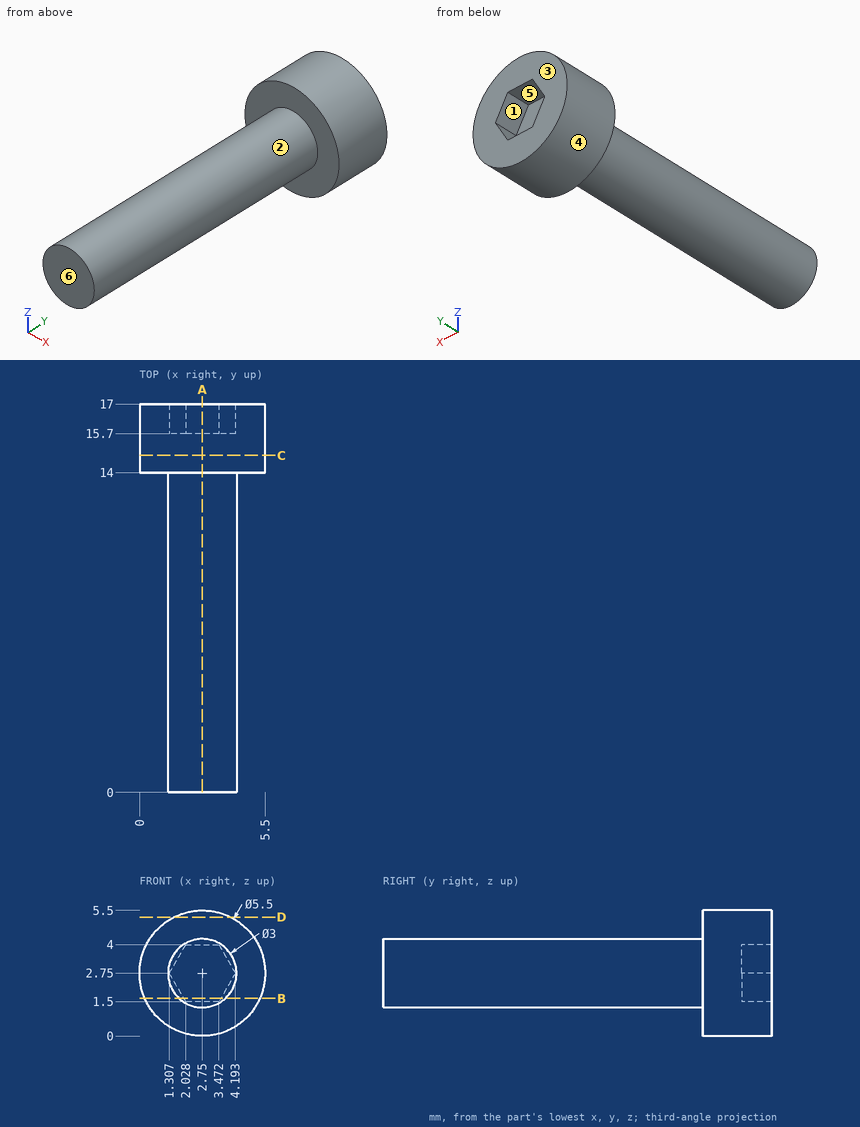
Answer from the drawing. Dimensions are ordinates in mm from the lowest x, y and z of the part. A direction names the side the tool comes from. Coordinates: 2 decimals unless noted, no trailing zeros. Order: outer loops, then holes, each group sorted by start corner. A loop starts at its lowest first (then second) coordinate and runs counter-clockwise, first axis right, second up. Notation, with made-up numbers: M -9.5,85 L 8.5,85 A24 ccw 8.5,122 Z; hole C 1.5,3.25 d10. An arc over 180 degrees is marked long. Put each result on its own line as item: value. Start each with the question number.
Item 1: For the marked faces 1, 2 and 3, determine the directions among +Z, -Z, +X, -X, +Y, -Y from which every point of the face is accessible in a straight line to the end or side of a thin tool.
Item 2: Section B-B, the plane z = 1.65 is taken. Determine the outline of the cut face in (x, y).
Item 3: Given pin 1 Ø1 at (y, z) = (10.5, 4) entering from -X; pin 2 Ø2 at (y, z) = (3, 1.5) entering from -X; pin 3 Ø3 at (x, z) = (2, 3) entering from +Y; pin 4 Ø1.5 at (x, y) = (3.5, 13.5) entering from -Z, each flat-ended and moving along its own axis, determine where each tip first touches the part or whether it passes through.
Item 4: Section D-D, the plane z = 5.2 is taken. Determine the outline of the cut face in (x, y).
Item 5: Section A-A, the plane x = 2.75 is taken. Determine the outline of the cut face in (y, z).
Item 6: Consider probe 1 along Y at (x, z) = (2.85, 3.1); probe 2 along Y at (x, z) = (4, 1.85); probe 3 along Z at (x, y) = (2.7, 12). Determine where each line is inside the solid, lowest interval first. Write a range as [from, to].
Item 7: Section C-C, the plane y = 14.75 is taken. Determine the outline of the cut face in (x, z).
Item 8: The mould has two halves that part along X. Classify the marked faces 4, 5 and 6: +X half, -X half, draft (parallel to the pull), parting line (faces both ways), or undercut.
Computed:
1. face 1: +Y
1. face 2: -Y
1. face 3: +Z, -Z, +X, -X, +Y
2. outline: M 0.23,14 L 1.73,14 L 1.73,0 L 3.77,0 L 3.77,14 L 5.27,14 L 5.27,17 L 3.56,17 L 3.56,15.7 L 1.94,15.7 L 1.94,17 L 0.23,17 Z
3. pin 1: stops at x = 1.45
3. pin 2: stops at x = 1.27
3. pin 3: stops at y = 17
3. pin 4: stops at z = 0.01
4. outline: M 1.5,14 L 4,14 L 4,17 L 1.5,17 Z
5. outline: M 0,1.25 L 14,1.25 L 14,0 L 17,0 L 17,1.5 L 15.7,1.5 L 15.7,4 L 17,4 L 17,5.5 L 14,5.5 L 14,4.25 L 0,4.25 Z
6. probe 1: y = [0, 15.7]
6. probe 2: y = [14, 17]
6. probe 3: z = [1.25, 4.25]
7. outline: C 2.75,2.75 d5.5
8. face 4: parting line
8. face 5: undercut
8. face 6: draft
